Check sheet for the modelled part. Datum: model origin and axes. Units: mm. Give positions to 0.01 mm unless a question says otherwise; leave off trailing zeros. Loops run counter-clockwise (first coordinate to the right, second up) from the corner with the lowest first, then second, coordinate; pieces in that order, holes last. Notation, with made-up numbers: (19.25, -33) - (31.25, -33) arc R9 ccw to (31.25, -28) - close; hole circle Ø2 at (-18.75, 74). An arc over 180 degrees is marked (long way). Answer in a Markdown table with one row per item. Add a question column.
(1) Sectioned sample at A-A on y = -0.5. Enter the section's corners in (x, z).
(2) Go/stop test with a flat-tipped pin: P1, Ø5.5, axis at x = -53.24, y = 37.28, coming from the +Z side. Record where the tip stops, or that it passes through.
(3) Sectioned sample at B-B on x = 48.5. Enter the section's corners in (y, z).
(4) Draft check along Y on faces 1 (the face through (-37.562, 55.377, 1.622)), 2 (the face through (-54.797, 54.486, 1.578)), 3 (the face through (54.797, -54.486, 1.578)). Enter one of: released by +Y, released by -Y, zero draft, split by the parting line, or undercut.
(5) Thickness scan on L1, parallel to X at y = -47, z = 0.8; L2, parallel to X at y = -53, z = 1.65; L3, parallel to Y at x = -48.5, z = 2.05. Record the ranges inside material, lowest first.
(6) Sectioned sample at C-C on z = 0.9. State how many separate pieces and enclosed holes the cut face has, then the cut area to 3 significant figures.
Autodesk Inventor part; units mm, degrees
ref_plane "YZ Plane" through (0, 0, 0) normal (1, 0, 0) x (0, 1, 0)
ref_plane "XZ Plane" through (0, 0, 0) normal (0, 1, 0) x (-1, 0, 0)
ref_plane "XY Plane" through (0, 0, 0) normal (0, 0, 1) x (1, 0, 0)
sketch "Sketch1" plane through (0, 0, 0) normal (0, 0, 1) x (1, 0, 0)
  circle A0 centre (0, 0) radius 57.5
  circle A1 centre (0, 0) radius 60.5
  line L0 (-40.5, 60.5) -> (40.5, 60.5)
  line L1 (60.5, 40.5) -> (60.5, -40.5)
  line L2 (40.5, -60.5) -> (-40.5, -60.5)
  line L3 (-60.5, -40.5) -> (-60.5, 40.5)
  arc A2 (-40.5, 60.5) -> (-60.5, 40.5) centre (-40.5, 40.5) ccw
  arc A3 (60.5, 40.5) -> (40.5, 60.5) centre (40.5, 40.5) ccw
  arc A4 (40.5, -60.5) -> (60.5, -40.5) centre (40.5, -40.5) ccw
  arc A5 (-60.5, -40.5) -> (-40.5, -60.5) centre (-40.5, -40.5) ccw
  dimension "d0" = 115
  dimension "d1" = 121
  dimension "d2" = 20
extrude "Extrusion1" add sketch "Sketch1" along normal blind 3.2
sketch "Sketch3" plane through (0, 0, 3.2) normal (0, 0, 1) x (1, 0, 0)
  circle A0 centre (-37.282468, -53.244883) radius 2.15
  circle A1 centre (-48.5, -48.5) radius 2.65
  circle A2 centre (-53.244883, -37.282468) radius 2.15
  circle A3 centre (-53.244883, 37.282468) radius 2.15
  circle A4 centre (-48.5, 48.5) radius 2.65
  circle A5 centre (-37.282468, 53.244883) radius 2.15
  circle A6 centre (37.282468, 53.244883) radius 2.15
  circle A7 centre (48.5, 48.5) radius 2.65
  circle A8 centre (53.244883, 37.282468) radius 2.15
  circle A9 centre (53.244883, -37.282468) radius 2.15
  circle A10 centre (48.5, -48.5) radius 2.65
  circle A11 centre (37.282468, -53.244883) radius 2.15
  point P0 (0, 0)
extrude "Extrusion3" cut sketch "Sketch3" against normal through all
sketch "Sketch4" plane through (0, 0, 3.2) normal (0, 0, 1) x (1, 0, 0)
  arc A0 (-52.049443, -21.979661) -> (-53.351667, -21.444104) centre (-52.970672, -22.368681) ccw
  arc A1 (-52.573656, -23.286493) -> (-52.049443, -21.979661) centre (-52.970672, -22.368681) ccw
  circle A2 centre (-52.970672, -22.368681) radius 0.95
  point P0 (0, 0)
  dimension "d28" = 1.9
extrude "Extrusion4" add sketch "Sketch4" against normal up to surface (3.2 mm away)
sketch "Sketch5" plane through (0, 0, 3.2) normal (0, 0, 1) x (1, 0, 0)
  arc A0 (-52.593886, -23.240766) -> (-53.332999, -21.49049) centre (0, 0) ccw
  circle A1 centre (0, 0) radius 57.55
  arc A2 (-52.593886, -23.240766) -> (-53.332999, -21.49049) centre (-52.970672, -22.368681) ccw
  line L0 (-52.593886, -23.240766) -> (-52.651569, -23.263484)
  line L1 (-53.332999, -21.49049) -> (-53.442689, -21.544242)
  point P0 (-52.640446, -23.259104)
  point P1 (-53.378017, -21.51255)
  dimension "d31" = 0.05
sketch "Sketch5 outline for Extrusion5" plane through (0, 0, 3.2) normal (0, 0, 1) x (1, 0, 0)
  arc A0 (-53.332999, -21.49049) -> (-52.593886, -23.240766) centre (0, 0) cw
  line L0 (-53.378017, -21.51255) -> (-53.332999, -21.49049)
  arc A1 (-52.640446, -23.259104) -> (-53.378017, -21.51255) centre (0, 0) ccw
  line L1 (-52.593886, -23.240766) -> (-52.640446, -23.259104)
extrude "Extrusion5" cut sketch "Sketch5 outline for Extrusion5" against normal through all
properties part number "stator_center_00_alu"
Reply:
| question | item | result |
|---|---|---|
| 1 | outline | (-60.5, 0) - (-57.55, 0) - (-57.55, 3.2) - (-60.5, 3.2) - close; (57.55, 0) - (60.5, 0) - (60.5, 3.2) - (57.55, 3.2) - close |
| 2 | P1 | z = 3.2 |
| 3 | outline | (-58.83, 0) - (-51.15, 0) - (-51.15, 3.2) - (-58.83, 3.2) - close; (-45.85, 0) - (-30.98, 0) - (-30.98, 3.2) - (-45.85, 3.2) - close; (30.98, 0) - (45.85, 0) - (45.85, 3.2) - (30.98, 3.2) - close; (51.15, 0) - (58.83, 0) - (58.83, 3.2) - (51.15, 3.2) - close |
| 4 | face 1 | undercut |
| 4 | face 2 | released by +Y |
| 4 | face 3 | released by -Y |
| 5 | L1 | -59.41 to -50.68, -46.32 to -33.21, 33.21 to 46.32, 50.68 to 59.41 |
| 5 | L2 | -56.11 to -39.42, -35.15 to -22.43, 22.43 to 35.15, 39.42 to 56.11 |
| 5 | L3 | -58.83 to -51.15, -45.85 to -30.98, 30.98 to 45.85, 51.15 to 58.83 |
| 6 | separate pieces | 1 |
| 6 | enclosed holes | 13 |
| 6 | area | 3,690 mm^2 |
